Autodesk Inventor part; units mm, degrees
ref_plane "YZ Plane" through (0, 0, 0) normal (1, 0, 0) x (0, 1, 0)
ref_plane "XZ Plane" through (0, 0, 0) normal (0, 1, 0) x (-1, 0, 0)
ref_plane "XY Plane" through (0, 0, 0) normal (0, 0, 1) x (1, 0, 0)
sketch "スケッチ1" plane through (0, 0, 0) normal (0, 1, 0) x (-1, 0, 0)
  line L0 (0, 0) -> (5, 0)
  line L1 (5, 0) -> (5, -65)
  line L2 (5, -65) -> (0, -65)
  line L3 (0, -65) -> (0, 0)
  dimension "d0" = 5
  dimension "d1" = 65
extrude "押し出し1" add sketch "スケッチ1" along normal blind 3
sketch "スケッチ2" plane through (0, 3, 0) normal (0, 1, 0) x (1, 0, 0)
  line L0 (-5, 0) -> (0, 0)
  line L1 (-5, 0) -> (0, 0)
  line L2 (0, 0) -> (0, 5)
  line L3 (0, 5) -> (-5, 5)
  line L4 (-5, 5) -> (-5, 0)
  line L5 (0, 65) -> (-5, 65)
  line L6 (-5, 65) -> (0, 65)
  line L7 (0, 65) -> (0, 60)
  line L8 (0, 60) -> (-5, 60)
  line L9 (-5, 60) -> (-5, 65)
  dimension "d4" = 5
  dimension "d5" = 5
  dimension "d6" = 5
  dimension "d7" = 5
extrude "押し出し2" add sketch "スケッチ2" along normal blind 3
sketch "スケッチ3" plane through (0, 6, 0) normal (0, 1, 0) x (1, 0, 0)
  line L0 (0, 60) -> (0, 65)
  line L1 (0, 65) -> (-5, 65)
  line L2 (-5, 0) -> (0, 0)
  point P0 (-2.5, 2.5)
  point P1 (-2.5, 62.5)
  dimension "d10" = 2.5
  dimension "d11" = 2.5
  dimension "d12" = 2.5
hole "穴1" at (-2.5, 6, -2.5) at (-2.5, 6, -62.5) direction (0, -1, 0) diameter 3.2 depth 5 tip angle 118
sketch "スケッチ4" plane through (0, 3, 0) normal (0, 1, 0) x (1, 0, 0)
  circle A0 centre (-2.5, 52.5) radius 1.6
  circle A1 centre (-2.5, 12.5) radius 1.6
  line L0 (0, 65) -> (-5, 65)
  line L1 (-5, 0) -> (0, 0)
  line L2 (-5, 60) -> (-5, 5)
  dimension "d20" = 3.2
  dimension "d21" = 3.2
  dimension "d22" = 40
  dimension "d23" = 12.5
  dimension "d24" = 12.5
  dimension "d25" = 2.5
extrude "押し出し3" add sketch "スケッチ4" along normal blind 3
properties part number "Tamiya-doubleGearBoxStopper"
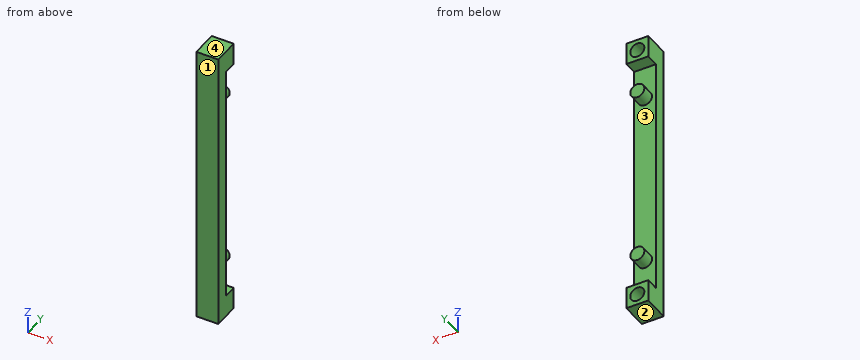
Part model, mm, in its own coordinate system. Face numbers are marked on the shaded views. Coordinates: 2 decimals unless noted, no trailing zeros. Write each loop counter-clockwise with the first axis right and the second up, starting at its lowest first coordinate (ties: lowest second). Pieces come first, ordered by that corner, then holes.
Item 1: Slice it at C-C (z = -25.5). Write the cut outline in (x, y), and give its area (3 significant figures).
Item 2: Pin check, flat tip, straight feed: pin 1 (2.5 mm diameter, centred on x = -2, z = -42, fed in from +Y). Stop position of the tip, or through.
Item 3: Mould opens along Z. For the marked faces 1, 2, 3 and 4 say: released by +Z, released by -Z, zero draft, split by the parting line, or undercut.
Item 4: Probe line 1 (Z direction, x = -2.5, y = 4); line 2 (Z direction, x = -2.5, y = 2.3); line 3 (X direction, y = 2.65, z = -2.5). List the from-to ranges inside material, lowest first.
Item 5: Slice it at A-A (y = 4.45). Write the cut outline in (x, z), and give its area (3 significant figures).
Item 6: Slice it at B-B (z = -12.5). Write the cut outline in (x, y), and give its area (3 significant figures).
Results found:
1. outline: (-5, 0) - (0, 0) - (0, 3) - (-5, 3) - close
1. area: 15.0 mm2
2. pin 1: stops at y = 3
3. face 1: zero draft
3. face 2: released by -Z
3. face 3: undercut
3. face 4: released by +Z
4. line 1: z = -65 to -64.1, -60.9 to -60, -54.1 to -50.9, -14.1 to -10.9, -5 to -4.1, -0.9 to 0
4. line 2: z = -65 to -64.1, -60.9 to -4.1, -0.9 to 0
4. line 3: x = -5 to -4.1, -0.9 to 0
5. outline: (-5, -65) - (0, -65) - (0, -60) - (-5, -60) - close; (-5, -5) - (0, -5) - (0, 0) - (-5, 0) - close; circle Ø3.2 at (-2.5, -52.5); circle Ø3.2 at (-2.5, -12.5); hole circle Ø3.2 at (-2.5, -62.5); hole circle Ø3.2 at (-2.5, -2.5)
5. area: 50.0 mm2
6. outline: (-5, 0) - (0, 0) - (0, 3) - (-0.9, 3) - (-0.9, 6) - (-4.1, 6) - (-4.1, 3) - (-5, 3) - close
6. area: 24.6 mm2
